Source: CAD feature listing. Evaluate the final solid. Frame: model axes, mm. A direction names the side the tool comes from. Give positions to 0.01 mm unless a question says otherwise; leave off trailing zeros. Order: outer loops, then holes, each group sorted by start corner. A loop starts at its lowest first (then second) coordinate and runs counter-clockwise, first axis right, second up. Notation, with made-up numbers: (-31.5, 30) -> (-2.5, 30) arc R21 cw to (-2.5, 38) -> close; hole circle Ø11 at (89.25, 69). An arc over 180 degrees is marked (long way). Answer in a Markdown table with one row per item.
```python
from build123d import *

# Parameters (mm, degrees)
F1_DEPTH = 12.5
F2_R     = 1.175
F3_DEPTH = 3
F4_W     = 15
F4_H     = 15
F5_DEPTH = 2.5
F6_W     = 12
F6_H     = 15
F7_DEPTH = 4.5


with BuildPart() as f1:
    # F0 (on Right) → F1 (new body, symmetric)
    with BuildSketch(Plane.YZ):
        with BuildLine():
            Line((16.5, 0), (10.5, 0))
            ThreePointArc((10.5, 0), (0, -10.5), (-10.5, 0))
            Line((-10.5, 0), (-12.5, 0))
            Line((-12.5, 0), (-12.5, -18.566574))
            Line((-12.5, -18.566574), (-1.889947, -18.566574))
            Line((-1.889947, -18.566574), (16.5, -18.566574))
            Line((16.5, -18.566574), (16.5, 0))
        make_face()
        with BuildLine():
            ThreePointArc((-10.5, 0), (0, 10.5), (10.5, 0))
            Line((10.5, 0), (16.5, 0))
            Line((16.5, 0), (16.5, 19.05242))
            Line((16.5, 19.05242), (-12.5, 19.05242))
            Line((-12.5, 19.05242), (-12.5, 0))
            Line((-12.5, 0), (-10.5, 0))
        make_face()
    extrude(amount=F1_DEPTH, both=True)

    # F2 (on face) → F3 (join)
    with BuildSketch(Plane.XY.offset(19.05242)):
        with Locations((-7.62, -9.7155)):
            Circle(F2_R)
        with BuildLine():
            ThreePointArc((7.62, -8.5405), (6.78915, -10.54635), (8.795, -9.7155))
            ThreePointArc((8.795, -9.7155), (8.45085, -8.88465), (7.62, -8.5405))
        make_face()
        with BuildLine():
            ThreePointArc((8.795, 11.8745), (6.78915, 12.70535), (7.62, 10.6995))
            ThreePointArc((7.62, 10.6995), (8.45085, 11.04365), (8.795, 11.8745))
        make_face()
        with Locations((-7.62, 11.8745)):
            Circle(F2_R)
    extrude(amount=F3_DEPTH)

    # F4 (on face) → F5 (cut)
    with BuildSketch(Plane(origin=(0, 0, -18.566574), x_dir=(1, 0, 0), z_dir=(0, 0, -1))):
        with Locations((0.837269, 0)):
            Rectangle(F4_W, F4_H)
    extrude(amount=-F5_DEPTH, mode=Mode.SUBTRACT)

    # F6 (on face) → F7 (cut)
    with BuildSketch(Plane(origin=(0, 16.5, 0), x_dir=(-1, 0, 0), z_dir=(0, 1, 0))):
        with Locations((0.127016, -1.779968)):
            Rectangle(F6_W, F6_H)
    extrude(amount=-F7_DEPTH, mode=Mode.SUBTRACT)


solid = f1.part
```
(1) Section query A-A (y = 0). Return the cut outline in (x, z).
A:
| item | result |
|---|---|
| outline | (-12.5, -18.57) -> (-6.66, -18.57) -> (-6.66, -16.07) -> (8.34, -16.07) -> (8.34, -18.57) -> (12.5, -18.57) -> (12.5, -10.5) -> (-12.5, -10.5) -> close; (-12.5, 10.5) -> (12.5, 10.5) -> (12.5, 19.05) -> (-12.5, 19.05) -> close |
(2) First-contact query: pin 1 Ø4 at (x, y) = (-4.5, -3) entering from +Z; pin 2 Ø2 at (y, z) = (-3, -9.5) entering from +X; pin 3 Ø7.5 at (x, y) = (1, 3) entering from -Z; pin 4 Ø1 at (x, z) = (2, -6.5) entering from +Y. Flat tips, straight axial feed; report the tip coordinate or a pass-through.
A:
| item | result |
|---|---|
| pin 1 | stops at z = 19.05 |
| pin 2 | stops at x = 12.5 |
| pin 3 | stops at z = -16.07 |
| pin 4 | stops at y = 12 |
(3) Section query D-D (x = -7.62). Return the cut outline in (y, z), plus the area to 3 significant figures.
A:
| item | result |
|---|---|
| outline | (-12.5, -18.57) -> (16.5, -18.57) -> (16.5, 19.05) -> (13.05, 19.05) -> (13.05, 22.05) -> (10.7, 22.05) -> (10.7, 19.05) -> (-8.54, 19.05) -> (-8.54, 22.05) -> (-10.89, 22.05) -> (-10.89, 19.05) -> (-12.5, 19.05) -> close; hole circle Ø21 at (0, 0) |
| area | 759 mm^2 |
(4) Pull-direction query (X, two-part tool) for faces 1 (the cylindrical face through (-8.794, -9.664, 20.531)), 2 (the flat face through (8, 12, 22.052)); classes: +X half, -X half, draft (parallel to the pull), parting line (faces both ways), or undercut.
A:
| item | result |
|---|---|
| face 1 | undercut |
| face 2 | draft |
(5) Section query C-C (x = 2.25). Return the cut outline in (y, z).
A:
| item | result |
|---|---|
| outline | (-12.5, -18.57) -> (-7.5, -18.57) -> (-7.5, -16.07) -> (7.5, -16.07) -> (7.5, -18.57) -> (16.5, -18.57) -> (16.5, -9.28) -> (12, -9.28) -> (12, 5.72) -> (16.5, 5.72) -> (16.5, 19.05) -> (-12.5, 19.05) -> close; hole circle Ø21 at (0, 0) |
(6) Section query B-B (z = 0). Return the cut outline in (x, y), plus the area to 3 significant figures.
A:
| item | result |
|---|---|
| outline | (-12.5, -12.5) -> (12.5, -12.5) -> (12.5, -10.5) -> (-12.5, -10.5) -> close; (-12.5, 10.5) -> (12.5, 10.5) -> (12.5, 16.5) -> (5.87, 16.5) -> (5.87, 12) -> (-6.13, 12) -> (-6.13, 16.5) -> (-12.5, 16.5) -> close |
| area | 146 mm^2 |
(7) Access query for faces 3 (the cylindrical face through (-8.794, 11.926, 20.531)), 4 (the flat face through (-6.663, 0, -17)), 5 (the flat face through (0, 14, 5.72)). Directions: +Z, -Z, +X, -X, +Y, -Y. A direction counts if a zero-diameter tool reaches every point of the face in a straight line with its end or side. Return the directions, or none.
A:
| item | result |
|---|---|
| face 3 | +Z |
| face 4 | -Z |
| face 5 | +Y |
(8) Ray query, probe 1 along Z at (x, y) = (3.5, 0); probe 2 along Y at (x, z) = (-8.5, -5); probe 3 along Y at (x, z) = (0, 9.5). Return the intervals inside material, ascending.
A:
| item | result |
|---|---|
| probe 1 | z = -16.07 to -10.5, 10.5 to 19.05 |
| probe 2 | y = -12.5 to -9.23, 9.23 to 16.5 |
| probe 3 | y = -12.5 to -4.47, 4.47 to 16.5 |
